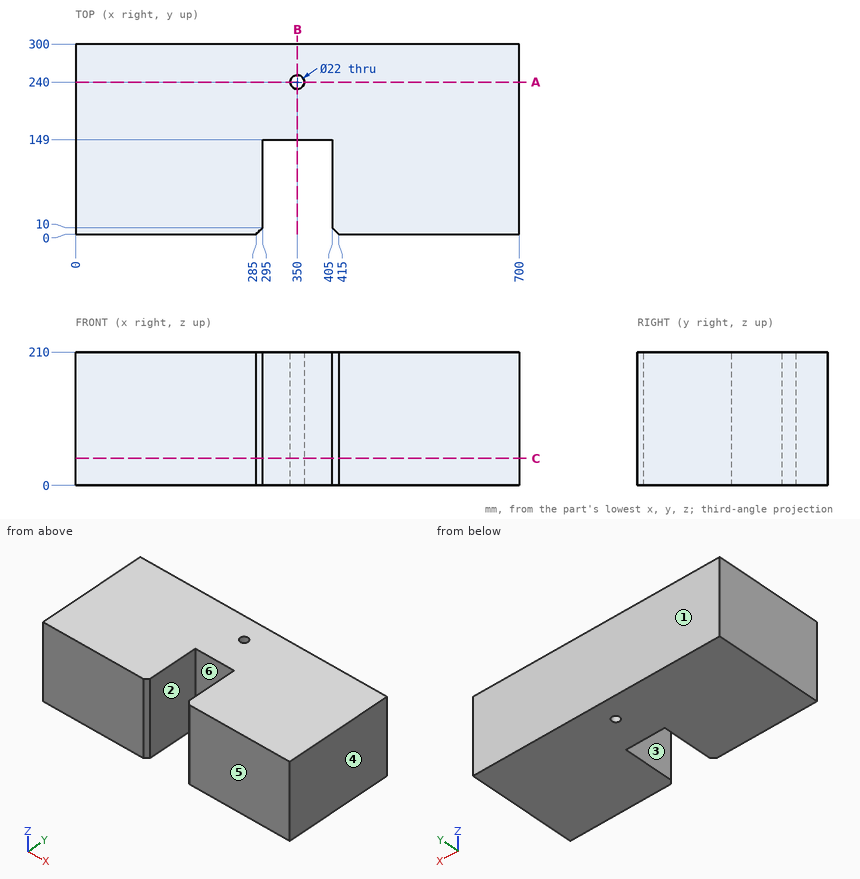
Geometry check sheet. Reference: drawing and pictorial views, mm from the part's lowest x, y, z. A direction names the side the tool comes from. Give positions to 0.01 mm unless a question says otherwise; leave off trailing zeros. Loops run counter-clockwise (first coordinate to the right, second up) from the corner with the lowest first, then second, coordinate; pieces in that order, holes last.
1. Mould release check, pull along X, two halves, no side actions. Record for the marked faces 3, 4, 5 and 6: released by +X, released by -X, zero draft, split by the parting line, or undercut.
2. Section check A-A, the plane y = 240. Enter the section's corners in (x, z), then the cut area to 3 significant figures.
3. Section check B-B, the plane x = 350. Enter the section's corners in (y, z), then the cut area to 3 significant figures.
4. Go/stop test with a flat-tipped pin: pin 1 Ø8 at (x, z) = (348.5, 128.5) entering from -Y. Record where the tip stops, or that it passes through.
5. Section check C-C, the plane z = 42.5. Enter the section's corners in (x, y), then the cut area to 3 significant figures.
6. Set-up check for the marked faces 1 and 2: record each of +Z, -Z, +X, -X, +Y, -Y from which the full face is reachable in a straight line by a thin tool's end or side.
7. Thickness scan on line 1 (X direction, y = 240, z = 145.5); line 2 (X direction, y = 28, z = 104.5); line 3 (Y direction, x = 350, z = 126). Record the ranges inside material, lowest first.
Geometry says:
1. face 3: undercut
1. face 4: released by +X
1. face 5: zero draft
1. face 6: undercut
2. outline: (0, 0) - (339, 0) - (339, 210) - (0, 210) - close; (361, 0) - (700, 0) - (700, 210) - (361, 210) - close
2. area: 142,000 mm2
3. outline: (149, 0) - (229, 0) - (229, 210) - (149, 210) - close; (251, 0) - (300, 0) - (300, 210) - (251, 210) - close
3. area: 27,100 mm2
4. pin 1: stops at y = 149
5. outline: (0, 0) - (285, 0) - (295, 10) - (295, 149) - (405, 149) - (405, 10) - (415, 0) - (700, 0) - (700, 300) - (0, 300) - close; hole circle Ø22 at (350, 240)
5. area: 193,000 mm2
6. face 1: +Z, -Z, +X, -X, +Y
6. face 2: +Z, -Z, -Y
7. line 1: x = 0 to 339, 361 to 700
7. line 2: x = 0 to 295, 405 to 700
7. line 3: y = 149 to 229, 251 to 300
